Here's how the part is built. I have some questions about the finished solid (model axes, mm). Face numbers are marked on the shaded views. Coordinates: 2 decimals unless noted, no trailing zeros. Write each loop counter-clockwise with the first axis right and the second up, starting at its lowest first coordinate (ties: lowest second). Pieces come first, ordered by that corner, then holes. Notation, with made-up numbers: M -5,4 L 32,4 A10 ccw 32,17 Z; hole C -20.75,-5 d4. An arc over 180 degrees is marked long. Write each question's results on one line, items separated by ' | '. Start each with the question number.
from build123d import *

# Parameters (mm, degrees)
FILLET1_R = 0.2


with BuildPart() as part:
    # Sketch1 → Revolve1 (revolve)
    with BuildSketch(Plane.XY):
        with BuildLine():
            Line((1.5875, -3.679795897), (1.5875, -6.985))
            Line((1.5875, -6.985), (1.7875, -6.985))
            Line((1.7875, -6.985), (1.7875, -3.679795897))
            ThreePointArc((1.7875, -3.679795897), (1.747091794, -3.279795897), (1.6275, -2.895959179))
            ThreePointArc((1.6275, -2.895959179), (1.597602051, -2.8), (1.5875, -2.7))
            Line((1.5875, -2.7), (1.5875, 0))
            Line((1.5875, 0), (3.175, 0))
            Line((3.175, 0), (3.175, 0.3))
            ThreePointArc((3.175, 0.3), (1.994886024, 0.767687303), (0.75, 1.016))
            Line((0.75, 1.016), (0.75, 0))
            Line((0.75, 0), (1.3875, 0))
            Line((1.3875, 0), (1.3875, -2.7))
            ThreePointArc((1.3875, -2.7), (1.401642872, -2.84), (1.4435, -2.974342851))
            ThreePointArc((1.4435, -2.974342851), (1.551132615, -3.319795897), (1.5875, -3.679795897))
        make_face()
    revolve(axis=Axis((0, 1.016, 0), (0, -1, 0)))

    # Fillet1
    fillet1_edges = [part.edges().sort_by_distance(p)[0] for p in [
        (-0.75, 1.016, 0),
    ]]
    fillet(fillet1_edges, radius=FILLET1_R)


solid = part.part
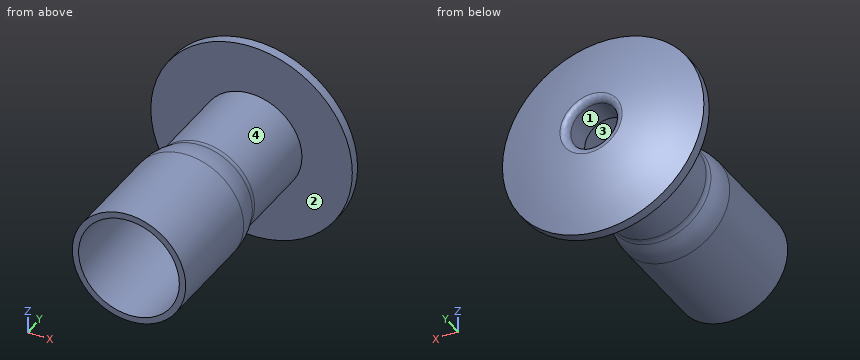
1) Please list where these lines run through material, in increasing order: line 1 (Z direction, x = 0, y = -0.85); line 2 (Z direction, x = 0, y = -5.9); line 3 (X direction, y = -3.5, z = 0.5). Write a range as [from, to].
2) We'd pull the mould along X, two halves only. Please class the marked faces 1, 2, 3 and 4: pulls with the +X half, pulls with the -X half, needs draft (parallel to the pull), parting line crosses it, or undercut.
3) I want a section at D-D, the plane y = -2.5. Write out the boundary of the cut face in (x, z) (1 decimal), then the cut area to 3 significant figures.
4) I want a section at B-B, the plane x = 2.5. Write out the boundary of the cut face in (y, z).
5) I want a section at A-A, the plane y = -5. Write out the boundary of the cut face in (x, z) (1 decimal).
6) For pin 1 Ø1.5 at (y, z) = (-5, -1) entering from +X, with a flat end and sliding along its axis, tell me the tip position at first contact or that it passes through.
7) I want a section at C-C, the plane z = -2.5. Write out the boundary of the cut face in (x, y), then the cut area to 3 significant figures.
Output:
1) line 1: z = [-1.59, -1.39], [1.39, 1.59] | line 2: z = [-1.79, -1.59], [1.59, 1.79] | line 3: x = [-1.71, -1.5], [1.5, 1.71]
2) face 1: undercut | face 2: needs draft | face 3: undercut | face 4: parting line crosses it
3) outline: C 0,0 d3.2; hole C 0,0 d2.8 | area: 1.87 mm2
4) outline: M 0,-1.96 L 0.3,-1.96 A6.59 ccw 0.3,1.96 L 0,1.96 Z
5) outline: C 0,0 d3.6; hole C 0,0 d3.2
6) pin 1: stops at x = 1.77
7) outline: M -1.96,0 L 1.96,0 L 1.96,0.3 A6.59 ccw -1.96,0.3 Z | area: 1.95 mm2
